Drawing for the job (mm, zero at the part's lowest x, y, z). Round coordinates to 2 decimals unless told otherwise and drop trailing zeros. Loops run counter-clockwise (first coordinate to the right, second up) from the corner with the lowest first, then second, coordinate; pieces in that order, holes last. Notation, with made-up numbers: (84, 63.5) - (108, 63.5) arc R17 ccw to (108, 91.5) - close; hole circle Ø5 at (-37, 76). An arc over 180 degrees is marked (long way). Put each result on its own line as item: value.
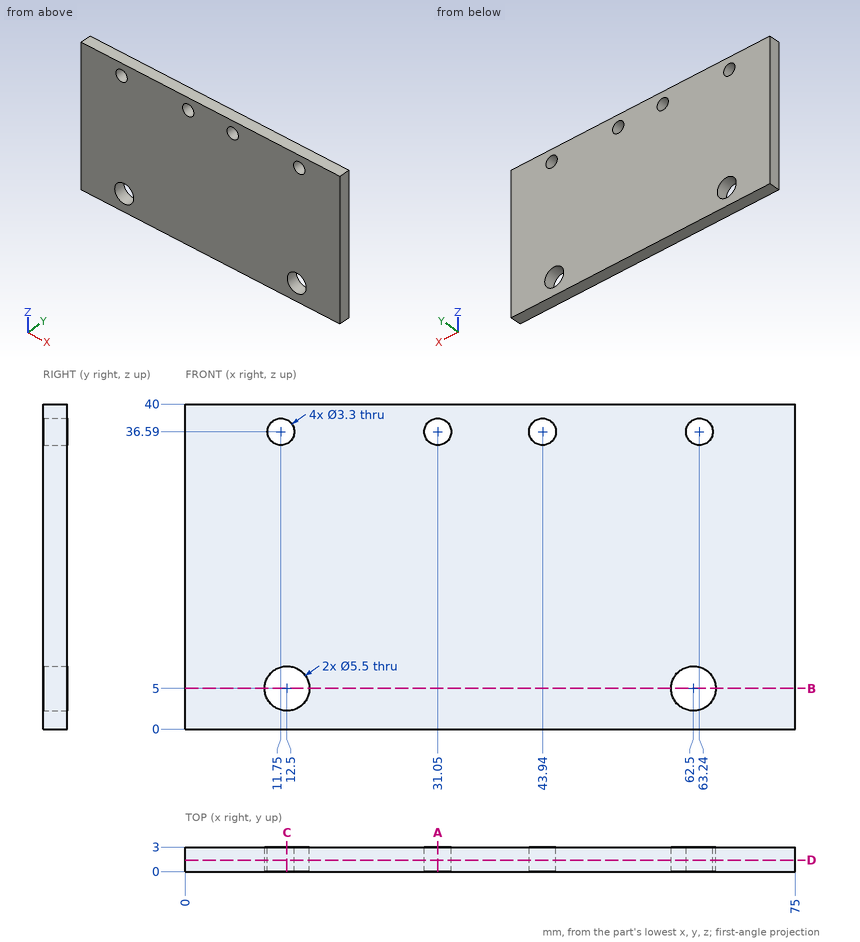
1. Band-saw the part on D-D (y = 1.4). List the corners of the cut face in (x, z), plus the area to 3 significant figures.
A:
outline: (0, 0) - (75, 0) - (75, 40) - (0, 40) - close; hole circle Ø5.5 at (12.5, 5); hole circle Ø3.3 at (11.75, 36.59); hole circle Ø3.3 at (31.05, 36.59); hole circle Ø3.3 at (43.94, 36.59); hole circle Ø5.5 at (62.5, 5); hole circle Ø3.3 at (63.24, 36.59)
area: 2,920 mm²
2. Probe line 1 along Z through (x, y) = (31.05, 1.3); line 2 along Z through (x, y) = (12.5, 0.7); line 3 along Z through (x, y) = (63.24, 1.6). List the from-to ranges inside material, lowest first. Write a range as [from, to].
A:
line 1: z = [0, 34.94], [38.24, 40]
line 2: z = [0, 2.25], [7.75, 35.12], [38.06, 40]
line 3: z = [0, 2.35], [7.65, 34.94], [38.24, 40]
3. Band-saw the part on A-A (x = 31.05). List the corners of the cut face in (y, z), plus the area to 3 significant figures.
A:
outline: (0, 0) - (3, 0) - (3, 34.94) - (0, 34.94) - close; (0, 38.24) - (3, 38.24) - (3, 40) - (0, 40) - close
area: 110 mm²
4. Band-saw the part on C-C (x = 12.5). List the corners of the cut face in (y, z).
A:
outline: (0, 0) - (3, 0) - (3, 2.25) - (0, 2.25) - close; (0, 7.75) - (3, 7.75) - (3, 35.12) - (0, 35.12) - close; (0, 38.06) - (3, 38.06) - (3, 40) - (0, 40) - close
5. Band-saw the part on B-B (z = 5). List the corners of the cut face in (x, y).
A:
outline: (0, 0) - (9.75, 0) - (9.75, 3) - (0, 3) - close; (15.25, 0) - (59.75, 0) - (59.75, 3) - (15.25, 3) - close; (65.25, 0) - (75, 0) - (75, 3) - (65.25, 3) - close
